```python
from build123d import *

# Parameters (mm, degrees)
F0_W     = 200
F0_H     = 1500
F0_W_2   = 10
F0_H_2   = 30
F1_DEPTH = 25
F2_DEPTH = 20


with BuildPart() as f1:
    # F0 (on Front) → F1 (new body)
    with BuildSketch(Plane.XZ):
        Rectangle(F0_W, F0_H)
        with Locations((-65, -172)):
            Rectangle(F0_W_2, F0_H_2, mode=Mode.SUBTRACT)
        with Locations((-65, -114.274818)):
            Rectangle(F0_W_2, F0_H_2, mode=Mode.SUBTRACT)
        with Locations((-65, -56.549635)):
            Rectangle(F0_W_2, F0_H_2, mode=Mode.SUBTRACT)
        with Locations((65, -172)):
            Rectangle(F0_W_2, F0_H_2, mode=Mode.SUBTRACT)
        with Locations((65, -114.274818)):
            Rectangle(F0_W_2, F0_H_2, mode=Mode.SUBTRACT)
        with Locations((65, -56.549635)):
            Rectangle(F0_W_2, F0_H_2, mode=Mode.SUBTRACT)
        with Locations((-65, 1.175547)):
            Rectangle(F0_W_2, F0_H_2, mode=Mode.SUBTRACT)
        with Locations((-65, 58.90073)):
            Rectangle(F0_W_2, F0_H_2, mode=Mode.SUBTRACT)
        with Locations((-65, 116.625912)):
            Rectangle(F0_W_2, F0_H_2, mode=Mode.SUBTRACT)
        with Locations((-65, 174.351094)):
            Rectangle(F0_W_2, F0_H_2, mode=Mode.SUBTRACT)
        with Locations((-65, 232.076277)):
            Rectangle(F0_W_2, F0_H_2, mode=Mode.SUBTRACT)
        with Locations((-65, 289.801459)):
            Rectangle(F0_W_2, F0_H_2, mode=Mode.SUBTRACT)
        with Locations((-65, 347.526642)):
            Rectangle(F0_W_2, F0_H_2, mode=Mode.SUBTRACT)
        with Locations((-65, 405.251824)):
            Rectangle(F0_W_2, F0_H_2, mode=Mode.SUBTRACT)
        with Locations((-65, 462.977007)):
            Rectangle(F0_W_2, F0_H_2, mode=Mode.SUBTRACT)
        with Locations((-65, 520.702189)):
            Rectangle(F0_W_2, F0_H_2, mode=Mode.SUBTRACT)
        Polygon((-56, -230), (-20, -230), (-20, 615.702189), (20, 615.702189), (20, -230), (56, -230), (56, -320), (-56, -320), align=None, mode=Mode.SUBTRACT)
        with Locations((65, 1.175547)):
            Rectangle(F0_W_2, F0_H_2, mode=Mode.SUBTRACT)
        with Locations((65, 58.90073)):
            Rectangle(F0_W_2, F0_H_2, mode=Mode.SUBTRACT)
        with Locations((65, 116.625912)):
            Rectangle(F0_W_2, F0_H_2, mode=Mode.SUBTRACT)
        with Locations((65, 174.351094)):
            Rectangle(F0_W_2, F0_H_2, mode=Mode.SUBTRACT)
        with Locations((65, 232.076277)):
            Rectangle(F0_W_2, F0_H_2, mode=Mode.SUBTRACT)
        with Locations((65, 289.801459)):
            Rectangle(F0_W_2, F0_H_2, mode=Mode.SUBTRACT)
        with Locations((65, 347.526642)):
            Rectangle(F0_W_2, F0_H_2, mode=Mode.SUBTRACT)
        with Locations((65, 405.251824)):
            Rectangle(F0_W_2, F0_H_2, mode=Mode.SUBTRACT)
        with Locations((65, 462.977007)):
            Rectangle(F0_W_2, F0_H_2, mode=Mode.SUBTRACT)
        with Locations((65, 520.702189)):
            Rectangle(F0_W_2, F0_H_2, mode=Mode.SUBTRACT)
    extrude(amount=F1_DEPTH)

    # F0 (on Front) → F2 (join)
    with BuildSketch(Plane.XZ):
        Polygon((-20, -265), (-20, -230), (-56, -230), (-56, -320), (56, -320), (56, -230), (20, -230), (20, -265), (48, -265), (48, -295), (-48, -295), (-48, -265), align=None)
    extrude(amount=F2_DEPTH)


solid = f1.part
```
The listing builds one solid part. Answer for the finished solid, in the listing's coordinates (mm). Coordinates: 2 decimals unless noted, no trailing zeros. Write each loop counter-clockwise with the first axis right and the second up, starting at its lowest first coordinate (ties: lowest second). Pieces come first, ordered by that corner, then holes. Notation, with made-up numbers: M 87,-11.75 L 145,-11.75 A29 ccw 145,14.25 Z; hole C 86.5,69.5 d3. An arc over 180 degrees is marked long. Use a Markdown table: item, result. Add a question column.
1. Section B-B (y = -11) is taken. Count the separate pieces of the cut face and the enclosed holes in it, plus the area to 3 significant figures.
2. For a pull along Z with two mould halves and no side action, classify faces 1 (the flat face through (-24, 0, 10)), 2 (the flat face through (70, -12, 463)) as +Z half, -Z half, draft (parallel to the pull), parting line (faces both ways), or undercut.
3. Section A-A (x = 0) is taken. Give the vertices of the cut face in (y, z).
4. Straight lines are drawn through the part: line 1 along Z through (x, y) = (-2.5, -5.75); line 2 along Z through (x, y) = (-43.5, -4.75); line 3 along X through (y, z) = (-5, 598.5). For each, find the intervals that lie inside material, in ascending order. Write a range as [from, to].
Data:
| question | item | result |
|---|---|---|
| 1 | separate pieces | 1 |
| 1 | enclosed holes | 27 |
| 1 | area | 254,000 mm2 |
| 2 | face 1 | draft |
| 2 | face 2 | undercut |
| 3 | outline | M -25,-750 L 0,-750 L 0,-295 L -20,-295 L -20,-320 L -25,-320 Z; M -25,615.7 L 0,615.7 L 0,750 L -25,750 Z |
| 4 | line 1 | z = [-750, -295], [615.7, 750] |
| 4 | line 2 | z = [-750, -295], [-265, 750] |
| 4 | line 3 | x = [-100, -20], [20, 100] |
